Source: three-view drawing plus pictorial views. Frame: mm from the lowest corner of the part. Give positions to 0.01 mm unless a question says otherwise; leave off trailing zeros. Write each loop counter-clockwise with the first axis right and the second up, starting at its lowest first coordinate (ties: lowest second). Pieces come first, ordered by that corner, then holes.
Q1. Cut plane B-B on x = 140. Return the cut outline in (y, z), plus the area to 4 significant figures.
Q2. Cut plane C-C on x = 50. Return the cut outline in (y, z), plus the area to 3 significant figures.
Q3. Pin query (flat end, axial travel): pin 1 (4.5 mm diameter, centred on x = 10, z = 30, fed in from -Y). Return the tip coordinate at first contact, or that it passes through.
Q4. Cut plane A-A on z = 30. Return the cut outline in (x, y), plus the area to 3 significant figures.
Q5. Line query: L1, parallel to X at y = 7, z = 30; L2, parallel to Z at x = 140, y = 8.25; L3, parallel to X at y = 9.5, z = 15. Output: solid intervals per line, ascending.
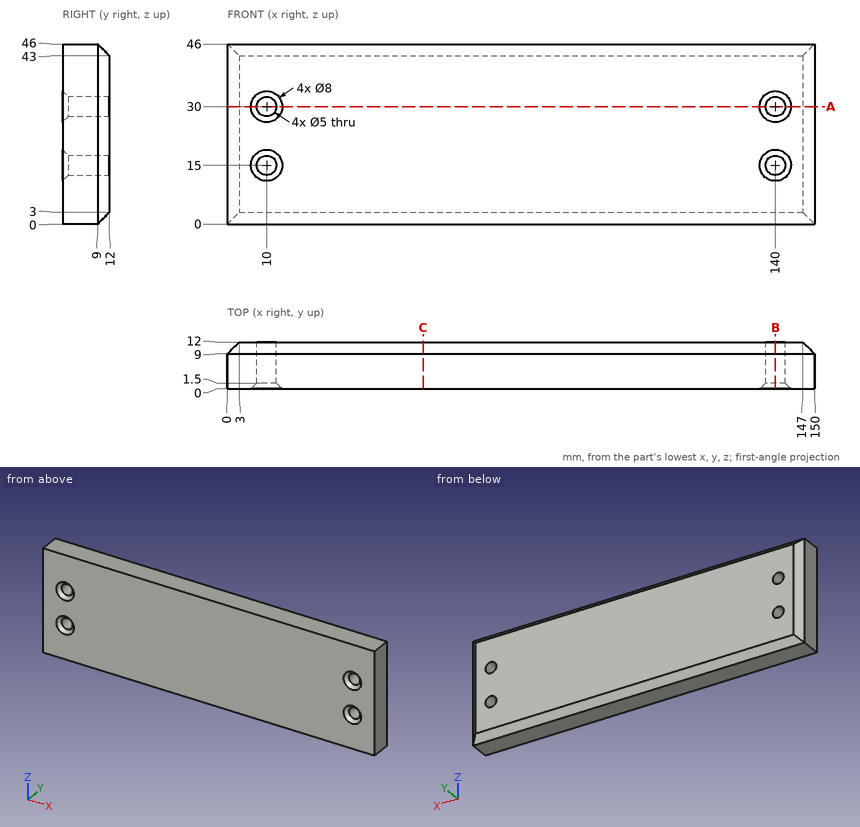
Data:
1. outline: (0, 0) - (9, 0) - (12, 3) - (12, 12.5) - (1.5, 12.5) - (0, 11) - close; (0, 19) - (1.5, 17.5) - (12, 17.5) - (12, 27.5) - (1.5, 27.5) - (0, 26) - close; (0, 34) - (1.5, 32.5) - (12, 32.5) - (12, 43) - (9, 46) - (0, 46) - close
1. area: 418.5 mm2
2. outline: (0, 0) - (9, 0) - (12, 3) - (12, 43) - (9, 46) - (0, 46) - close
2. area: 543 mm2
3. pin 1: passes through
4. outline: (0, 0) - (6, 0) - (7.5, 1.5) - (7.5, 12) - (3, 12) - (0, 9) - close; (12.5, 1.5) - (14, 0) - (136, 0) - (137.5, 1.5) - (137.5, 12) - (12.5, 12) - close; (142.5, 1.5) - (144, 0) - (150, 0) - (150, 9) - (147, 12) - (142.5, 12) - close
4. area: 1,670 mm2
5. L1: x = 0 to 7.5, 12.5 to 137.5, 142.5 to 150
5. L2: z = 0 to 12.5, 17.5 to 27.5, 32.5 to 46
5. L3: x = 0.5 to 7.5, 12.5 to 137.5, 142.5 to 149.5
